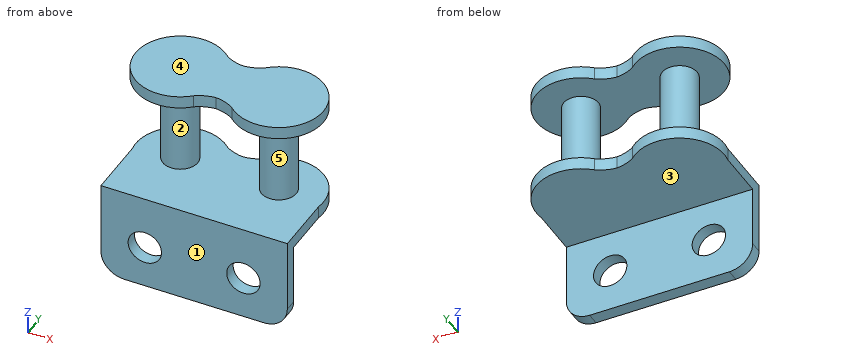
from build123d import *

# Parameters (mm, degrees)
SKETCH_1_R          = 4.25
SKETCH_1_R_2        = 2.25
EXTRUDE_1_DEPTH     = 4.45
EXTRUDE_1_2_DEPTH   = 4.45
SKETCH_2_R          = 5.75
SKETCH_2_R_2        = 4.25
SKETCH_2_R_3        = 2.25
EXTRUDE_3_DEPTH     = 1.6
SKETCH_3_R          = 4.25
CUT_EXTRUDE_1_DEPTH = 4.45
EXTRUDE_START       = -13.1
SKETCH_4_R          = 2.25
EXTRUDE_4_DEPTH     = 13.1
EXTRUDE_START_2     = 1.6
SKETCH_5_W          = 24
SKETCH_5_H          = 7.832292175
EXTRUDE_6_DEPTH     = 1.6
SKETCH_6_W          = 24
SKETCH_6_H          = 1.6
EXTRUDE_7_DEPTH     = 10.85
SKETCH_9_R          = 2.15
CUT_EXTRUDE_2_DEPTH = 28.22650373
FILLET_1_R          = 3


with BuildPart() as part:
    # Sketch 1 → Extrude 1 (new body)
    with BuildSketch(Plane.XY):
        with Locations((-6.35, 0)):
            Circle(SKETCH_1_R)
        with Locations((-6.35, 0)):
            Circle(SKETCH_1_R_2, mode=Mode.SUBTRACT)
    extrude(amount=EXTRUDE_1_DEPTH)



with BuildPart() as body_2:
    # Sketch 1 → Extrude 1 2 (new body)
    with BuildSketch(Plane.XY):
        with Locations(Location((6.35, 0, 0), (0, 0, 180))):
            Circle(SKETCH_1_R)
        with Locations(Location((6.35, 0, 0), (0, 0, 180))):
            Circle(SKETCH_1_R_2, mode=Mode.SUBTRACT)
    extrude(amount=EXTRUDE_1_2_DEPTH)


with BuildPart() as part_1:
    add(part.part)

    add(body_2.part)  # Extrude 3 merges body 2
    # Sketch 2 → Extrude 3 (add)
    # profile 1 of 4: a face of its own
    with BuildSketch(Plane.XY.offset(4.45)):
        with Locations((-6.35, 0)):
            Circle(SKETCH_2_R)
        with Locations((-6.35, 0)):
            Circle(SKETCH_2_R_2, mode=Mode.SUBTRACT)
    # profile 2 of 4: a face of its own
    with BuildSketch(Plane.XY.offset(4.45)):
        with Locations((-6.35, 0)):
            Circle(SKETCH_2_R_2)
        with Locations((-6.35, 0)):
            Circle(SKETCH_2_R_3, mode=Mode.SUBTRACT)
    # profile 3 of 4: a face of its own
    with BuildSketch(Plane.XY.offset(4.45)):
        with BuildLine():
            ThreePointArc((-2.464522189, 4.238580208), (-1.086731177, 2.315275641), (-0.6, 0))
            ThreePointArc((-0.6, 0), (-1.086731177, -2.315275641), (-2.464522189, -4.238580208))
            add(Edge.make_bspline(
                [(-2.464522189, -4.238580208), (-1.801147303, -3.67793909), (-0.370790644, -3.34588107), (0, -3.386350938)],
                knots=[0, 0, 0, 0, 1, 1, 1, 1], degree=3))
            add(Edge.make_bspline(
                [(2.464522189, -4.238580208), (1.801147303, -3.67793909), (0.370790644, -3.34588107), (0, -3.386350938)],
                knots=[0, 0, 0, 0, 1, 1, 1, 1], degree=3))
            ThreePointArc((2.464522189, -4.238580208), (0.6, 0), (2.464522189, 4.238580208))
            add(Edge.make_bspline(
                [(2.464522189, 4.238580208), (1.801147303, 3.67793909), (0.370790644, 3.34588107), (0, 3.386350938)],
                knots=[0, 0, 0, 0, 1, 1, 1, 1], degree=3))
            add(Edge.make_bspline(
                [(-2.464522189, 4.238580208), (-1.801147303, 3.67793909), (-0.370790644, 3.34588107), (0, 3.386350938)],
                knots=[0, 0, 0, 0, 1, 1, 1, 1], degree=3))
        make_face()
    # profile 4 of 4: a face of its own
    with BuildSketch(Plane.XY.offset(4.45)):
        with Locations((6.35, 0)):
            Circle(SKETCH_2_R)
        with Locations(Location((6.35, 0, 0), (0, 0, 180))):
            Circle(SKETCH_2_R_3, mode=Mode.SUBTRACT)
    extrude(amount=EXTRUDE_3_DEPTH)

    # Sketch 3 → Cut-Extrude 1 (cut)
    with BuildSketch(Plane(origin=(0, 0, 0), x_dir=(-1, 0, 0), z_dir=(0, 0, -1))):
        with Locations((6.35, 0)):
            Circle(SKETCH_3_R)
        with Locations((-6.35, 0)):
            Circle(SKETCH_3_R)
    extrude(amount=-CUT_EXTRUDE_1_DEPTH, mode=Mode.SUBTRACT)

    # Sketch 4 → Extrude 4 (add)
    with BuildSketch(Plane.XY.offset(6.05).offset(EXTRUDE_START)):
        with Locations((-6.35, 0)):
            Circle(SKETCH_4_R)
        with Locations((6.35, 0)):
            Circle(SKETCH_4_R)
    extrude(amount=EXTRUDE_4_DEPTH)

    # Sketch 5 → Extrude 6 (add)
    with BuildSketch(Plane(origin=(0, 0, -7.05), x_dir=(-1, 0, 0), z_dir=(0, 0, -1)).offset(EXTRUDE_START_2)):
        with Locations((0, -4.983853912)):
            Rectangle(SKETCH_5_W, SKETCH_5_H)
        with BuildLine():
            ThreePointArc((2.464522189, -4.238580208), (12.1, 0), (2.464522189, 4.238580208))
            add(Edge.make_bspline(
                [(2.464522189, 4.238580208), (1.801147303, 3.67793909), (0.370790644, 3.34588107), (0, 3.386350938)],
                knots=[0, 0, 0, 0, 1, 1, 1, 1], degree=3))
            add(Edge.make_bspline(
                [(0, 3.386350938), (-0.370790644, 3.34588107), (-1.801147303, 3.67793909), (-2.464522189, 4.238580208)],
                knots=[0, 0, 0, 0, 1, 1, 1, 1], degree=3))
            ThreePointArc((-2.464522189, 4.238580208), (-12.1, 0), (-2.464522189, -4.238580208))
            add(Edge.make_bspline(
                [(-2.464522189, -4.238580208), (-1.801147303, -3.67793909), (-0.370790644, -3.34588107), (0, -3.386350938)],
                knots=[0, 0, 0, 0, 1, 1, 1, 1], degree=3))
            add(Edge.make_bspline(
                [(0, -3.386350938), (0.370790644, -3.34588107), (1.801147303, -3.67793909), (2.464522189, -4.238580208)],
                knots=[0, 0, 0, 0, 1, 1, 1, 1], degree=3))
        make_face()
    extrude(amount=-EXTRUDE_6_DEPTH)

    # Sketch 6 → Extrude 7 (add)
    with BuildSketch(Plane(origin=(0, 0, -8.65), x_dir=(-1, 0, 0), z_dir=(0, 0, -1))):
        with Locations((0, -8.1)):
            Rectangle(SKETCH_6_W, SKETCH_6_H)
    extrude(amount=EXTRUDE_7_DEPTH)

    # Sketch 9 → Cut-Extrude 2 (cut, through all)
    with BuildSketch(Plane.XZ.offset(8.9)):
        with Locations(Location((-6.35, -14, 0), (0, 0, 270))):
            Circle(SKETCH_9_R)
        with Locations((6.35, -14)):
            Circle(SKETCH_9_R)
    extrude(amount=-CUT_EXTRUDE_2_DEPTH, mode=Mode.SUBTRACT)

    # Fillet 1
    fillet_1_edges = [part_1.edges().sort_by_distance(p)[0] for p in [
        (-12, -8.1, -19.5),
        (12, -8.1, -19.5),
    ]]
    fillet(fillet_1_edges, radius=FILLET_1_R)


solid = part_1.part
Geometry check sheet. Reference: the model listing, model coordinates, mm. Face numbers are marked on the shaded views. A direction names the side the tool comes from. Give positions to 0.01 mm unless a question says otherwise; leave off trailing zeros. Order: outer loops, then holes, each group sorted by start corner. A loop starts at its lowest first (then second) coordinate and runs counter-clockwise, first axis right, second up. Notation, with made-up numbers: (89, 38) - (93, 38) arc R34 cw to (93, 71) - close; hole circle Ø5 at (36, 88). An arc over 180 degrees is marked (long way). Answer as a JSON object with one key per item and string values.
(1) Draft check along X on the marked faces 4 and 5. Enter one of: released by +X, released by -X, zero draft, split by the parting line, or undercut.
Report:
{"face 4": "zero draft", "face 5": "undercut"}
(2) Cross-section at D-D (y = -5.25). Record the cut outline in (x, z).
Report:
{"outline": "(-12, -8.65) - (12, -8.65) - (12, -7.05) - (-12, -7.05) - close; (-8.7, 4.45) - (-4, 4.45) - (-4, 6.05) - (-8.7, 6.05) - close; (4, 4.45) - (8.7, 4.45) - (8.7, 6.05) - (4, 6.05) - close"}
(3) Cross-section at C-C (y = 0). Record the cut outline in (x, z).
Report:
{"outline": "(-12.1, -8.65) - (12.1, -8.65) - (12.1, -7.05) - (8.6, -7.05) - (8.6, 4.45) - (12.1, 4.45) - (12.1, 6.05) - (-12.1, 6.05) - (-12.1, 4.45) - (-8.6, 4.45) - (-8.6, -7.05) - (-12.1, -7.05) - close; hole (-4.1, -7.05) - (4.1, -7.05) - (4.1, 4.45) - (-4.1, 4.45) - close"}
(4) Depth check by flat-ended pin: pin 1 Ø1.5 at (x, y) = (-8, 2.5) entering from -Z; pin 2 Ø5.5 at (x, z) = (-5.5, -15.5) entering from +Y; pin 3 Ø8.5 at (y, z) = (-4.5, -14) entering from -X; pin 4 Ø3.5 at (x, z) = (-6.35, -14) entering from -Y. Enter the tip coordinate at first touch or a pass-through.
Report:
{"pin 1": "z = -8.65", "pin 2": "y = -7.3", "pin 3": "x = -12", "pin 4": "through"}
(5) Cross-section at B-B (z = -14). Record the cut outline in (x, y).
Report:
{"outline": "(-12, -8.9) - (-8.5, -8.9) - (-8.5, -7.3) - (-12, -7.3) - close; (-4.2, -8.9) - (4.2, -8.9) - (4.2, -7.3) - (-4.2, -7.3) - close; (8.5, -8.9) - (12, -8.9) - (12, -7.3) - (8.5, -7.3) - close"}
(6) Cross-section at A-A (x = -6.35). Record the cut outline in (y, z), then the cut area to 3 significant figures.
Report:
{"outline": "(-8.9, -19.5) - (-7.3, -19.5) - (-7.3, -16.15) - (-8.9, -16.15) - close; (-8.9, -11.85) - (-7.3, -11.85) - (-7.3, -8.65) - (5.75, -8.65) - (5.75, -7.05) - (2.25, -7.05) - (2.25, 4.45) - (5.75, 4.45) - (5.75, 6.05) - (-5.75, 6.05) - (-5.75, 4.45) - (-2.25, 4.45) - (-2.25, -7.05) - (-8.9, -7.05) - close", "area": "104 mm^2"}
(7) Tool access check on the marked faces 1, 2 and 3. Record the directions out of +Z, -Z, +X, -X, +Y, -Y that give a thin tool (end or side, any length) a straight path to the whole face; none if there is none.
Report:
{"face 1": "+Z, -Z, +X, -X, -Y", "face 2": "none", "face 3": "-Z, +X, -X, +Y"}
(8) Material ranges on line 1 (Z direction, x = 6.35, y = -8.25); line 2 (Z direction, x = 3, y = 0.5); line 3 (Z direction, x = -8.5, y = -6), recorded low to high.
Report:
{"line 1": "-19.5 to -16.15, -11.85 to -7.05", "line 2": "-8.65 to -7.05, 4.45 to 6.05", "line 3": "-8.65 to -7.05"}
